from build123d import *

# Parameters (mm, degrees)
SKETCH1_R                                       = 200
BOSS_EXTRUDE1_DEPTH                             = 10
CSK_FOR_M5_FLAT_HEAD_MACHINE_SCREW1_D           = 5.5
CSK_FOR_M5_FLAT_HEAD_MACHINE_SCREW1_CSINK_D     = 10.4
CSK_FOR_M5_FLAT_HEAD_MACHINE_SCREW1_CSINK_ANGLE = 90
SHELL1_T                                        = 1.4
CSK_FOR_M5_FLAT_HEAD_MACHINE_SCREW2_D           = 5.5
CSK_FOR_M5_FLAT_HEAD_MACHINE_SCREW2_CSINK_D     = 10.4
CSK_FOR_M5_FLAT_HEAD_MACHINE_SCREW2_CSINK_ANGLE = 90


with BuildPart() as part:
    # Sketch1 → Boss-Extrude1 (new body)
    with BuildSketch(Plane(origin=(0, 0, 0), x_dir=(1, 0, 0), z_dir=(0, 1, 0))):
        with Locations(Location((0, 0, 0), (0, 0, 270))):
            Circle(SKETCH1_R)
    extrude(amount=BOSS_EXTRUDE1_DEPTH)

    # CSK for M5 Flat Head Machine Screw1 (through all)
    with Locations(Plane(origin=(0, 10, 0), x_dir=(1, 0, 0), z_dir=(0, 1, 0))):
        with Locations((-189.999966012, 0.113646638), (1.41743193, 189.994712786), (189.983382613, 2.512833264), (1.187924025, -189.996286376), (-133.812075975, -134.886353362), (-133.58256807, 135.113646638), (131.111481907, 137.512833264), (136.187924025, -132.487166736)):
            CounterSinkHole(CSK_FOR_M5_FLAT_HEAD_MACHINE_SCREW1_D / 2, CSK_FOR_M5_FLAT_HEAD_MACHINE_SCREW1_CSINK_D / 2, counter_sink_angle=CSK_FOR_M5_FLAT_HEAD_MACHINE_SCREW1_CSINK_ANGLE)

    # Shell1 (no face opened: a closed hollow body)
    add(offset(amount=-SHELL1_T, mode=Mode.PRIVATE), mode=Mode.SUBTRACT)

    # CSK for M5 Flat Head Machine Screw2 (through all)
    with Locations(Plane(origin=(0, 0, 0), x_dir=(-1, 0, 0), z_dir=(0, -1, 0))):
        with Locations((-80, 0), (-80, 55), (-80, -55), (80, 0), (80, 55), (80, -55)):
            CounterSinkHole(CSK_FOR_M5_FLAT_HEAD_MACHINE_SCREW2_D / 2, CSK_FOR_M5_FLAT_HEAD_MACHINE_SCREW2_CSINK_D / 2, counter_sink_angle=CSK_FOR_M5_FLAT_HEAD_MACHINE_SCREW2_CSINK_ANGLE)


solid = part.part
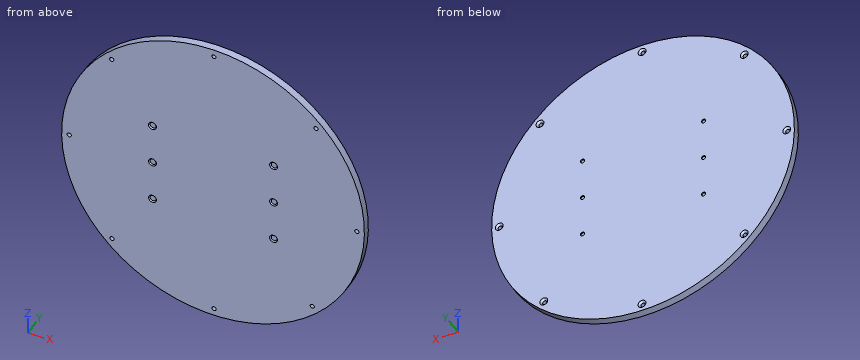
Model file for the job. Use its own axes, mm. Give positions to 0.01 mm unless a question says otherwise; leave off trailing zeros. Loops run counter-clockwise (first coordinate to the right, second up) from the corner with the lowest first, then second, coordinate; pieces in that order, holes last. Notation, with made-up numbers: (2, 3) -> (44, 3) arc R29 cw to (44, 34) -> close; hole circle Ø7 at (-10.75, 84.5). An arc over 180 degrees is marked (long way). Use a Markdown table: item, result. Add a question column.
(1) Slice it at C-C on z = 86.5. List the corners of the cut face in (x, y).
(2) Slice it at A-A on y = 3.75. Give the number of separate pieces and of enclosed holes in the cut face, and give its area (3 significant figures).
(3) Wall check: line 1 along Y through (x, z) = (-94.5, -43.5); line 2 along X through (y, z) = (9.45, 55); line 3 along Z through (x, y) = (-133, 2.5). Give the ranges that are in metal, low to high.
(4) Drop flat-ended pins along their axis: pin 1 Ø7 at (x, z) = (1.42, -189.99) entering from +Y; pin 2 Ø4 at (x, y) = (-27, 9) entering from +Z; pin 3 Ø3.5 at (x, z) = (-80, 0) entering from +Y; pin 4 Ø4 at (y, z) = (5.5, -59.5) entering from +X. Give the stop position or say it passes through.
(5) Slice it at B-B on x = 26. List the corners of the cut face in (y, z).
Filled sheet:
| question | item | result |
|---|---|---|
| 1 | outline | (-180.33, 0) -> (180.33, 0) -> (180.33, 10) -> (-180.33, 10) -> close; hole (-178.77, 1.4) -> (178.77, 1.4) -> (178.77, 8.6) -> (-178.77, 8.6) -> close |
| 2 | separate pieces | 9 |
| 2 | enclosed holes | 9 |
| 2 | area | 2,000 mm2 |
| 3 | line 1 | 0 to 1.4, 8.6 to 10 |
| 3 | line 2 | -192.29 to -82.75, -77.25 to 77.25, 82.75 to 192.29 |
| 3 | line 3 | -149.37 to -147.49, -139.22 to -137.8, -132.43 to -131, 130.82 to 132.26, 137.51 to 138.96, 147.49 to 149.37 |
| 4 | pin 1 | y = 8.31 |
| 4 | pin 2 | z = 198.43 |
| 4 | pin 3 | through |
| 4 | pin 4 | x = 191.56 |
| 5 | outline | (0, -198.3) -> (10, -198.3) -> (10, 198.3) -> (0, 198.3) -> close; hole (1.4, -196.89) -> (8.6, -196.89) -> (8.6, 196.89) -> (1.4, 196.89) -> close |
